The model under review builds one solid part; all positions refer to its coordinate system, in mm. Round coordinates to 2 decimals unless told otherwise and drop trailing zeros. Order: outer loops, then holes, each group sorted by start corner. A loop starts at its lowest first (then second) coordinate and runs counter-clockwise, first axis right, second up. Notation, with made-up numbers: M 19.5,79.5 L 64.5,79.5 A16 ccw 64.5,107.5 Z; hole C 35,-28.75 d3. An arc over 180 degrees is marked long. One line per item, written item: value. Start each with the question number.
from build123d import *

# Parameters (mm, degrees)
BOSS_EXTRUDE1_DEPTH = 3
SKETCH3_W           = 0.38
SKETCH3_H           = 0.38
BOSS_EXTRUDE2_DEPTH = 15


with BuildPart() as part:
    # PROF_TOP_VIEW → Boss-Extrude1 (new body)
    with BuildSketch(Plane(origin=(0, 0, 0), x_dir=(1, 0, 0), z_dir=(0, 1, 0))):
        Polygon((-2.03, 0), (2.03, 0), (2.03, -0.78499978), (1.27, -1.6), (-1.27, -1.6), (-2.03, -0.78499978), align=None)
    extrude(amount=-BOSS_EXTRUDE1_DEPTH)

    # Sketch3 → Boss-Extrude2 (add)
    with BuildSketch(Plane.XZ.offset(3)):
        with Locations((-1.27, 0.95)):
            Rectangle(SKETCH3_W, SKETCH3_H)
        with Locations((0, 0.95)):
            Rectangle(SKETCH3_W, SKETCH3_H)
        with Locations((1.27, 0.95)):
            Rectangle(SKETCH3_W, SKETCH3_H)
    extrude(amount=BOSS_EXTRUDE2_DEPTH)


solid = part.part
Item 1: Consider section D-D, the plane x = -0.7. Give the boundary of the cut face in (y, z), then the cut area to 3 significant figures.
Item 2: Consider section A-A, the plane y = -8. Give the boundary of the cut face in (x, z), then the cut area to 3 significant figures.
Item 3: Consider section C-C, the plane z = 0.25. Give the boundary of the cut face in (x, y), then the cut area to 3 significant figures.
Item 4: Consider section B-B, the plane x = 0. Give the boundary of the cut face in (y, z), then the cut area to 3 significant figures.
Item 5: Clearance check with a flat-ended pin moving along its axis: P1, Ø2, axis at x = 0, y = -5.5, coming from the -Z side. State where the tip first meets the part, or that it passes through.
Item 6: Wall thickness on L1, parallel to X at y = -4, z = 1.05; L2, parallel to Y at x = 0.7, z = 1; L3, parallel to Z at x = 1.4, y = -5.5: over which ranges is each line inside the solid? List them lowest first.
Computed:
1. outline: M -3,0 L 0,0 L 0,1.6 L -3,1.6 Z
1. area: 4.80 mm^2
2. outline: M -1.46,0.76 L -1.08,0.76 L -1.08,1.14 L -1.46,1.14 Z; M -0.19,0.76 L 0.19,0.76 L 0.19,1.14 L -0.19,1.14 Z; M 1.08,0.76 L 1.46,0.76 L 1.46,1.14 L 1.08,1.14 Z
2. area: 0.433 mm^2
3. outline: M -2.03,-3 L 2.03,-3 L 2.03,0 L -2.03,0 Z
3. area: 12.2 mm^2
4. outline: M -18,0.76 L -3,0.76 L -3,0 L 0,0 L 0,1.6 L -3,1.6 L -3,1.14 L -18,1.14 Z
4. area: 10.5 mm^2
5. P1: stops at z = 0.76
6. L1: x = -1.46 to -1.08, -0.19 to 0.19, 1.08 to 1.46
6. L2: y = -3 to 0
6. L3: z = 0.76 to 1.14
